from build123d import *

# Parameters (mm, degrees)
F0_R     = 16.6624
F1_DEPTH = 54.76875
F2_R     = 29.760102
F3_DEPTH = 20.6248
F4_R     = 11.1125
F5_DEPTH = 26.1874


with BuildPart() as f1:
    # F0 (on Top) → F1 (new body)
    with BuildSketch(Plane.XY):
        Circle(F0_R)
    extrude(amount=F1_DEPTH)

    # F2 (on face) → F3 (join)
    with BuildSketch(Plane(origin=(0, 0, 0), x_dir=(1, 0, 0), z_dir=(0, 0, -1))):
        Circle(F2_R)
    extrude(amount=F3_DEPTH)

    # F4 (on face) → F5 (join)
    with BuildSketch(Plane(origin=(0, 0, -20.6248), x_dir=(1, 0, 0), z_dir=(0, 0, -1))):
        Circle(F4_R)
    extrude(amount=F5_DEPTH)


solid = f1.part
Here's how the part is built. I have some questions about the finished solid (model axes, mm). A direction names the side the tool comes from. Round coordinates to 2 decimals unless told otherwise and drop trailing zeros. Order: outer loops, then holes, each group sorted by start corner. A loop starts at its lowest first (then second) coordinate and runs counter-clockwise, first axis right, second up. Notation, with made-up numbers: (8, -8) -> (21, -8) arc R21 cw to (21, 0) -> close; hole circle Ø1 at (0, 71.5). An arc over 180 degrees is marked (long way). Return JSON: item names as keys, results as strings.
Q1. If we section it at D-D on y = 13.5: List the corners of the cut face in (x, z) for me.
Filled sheet:
{"outline": "(-26.52, -20.62) -> (26.52, -20.62) -> (26.52, 0) -> (9.77, 0) -> (9.77, 54.77) -> (-9.77, 54.77) -> (-9.77, 0) -> (-26.52, 0) -> close"}
Q2. If we section it at A-A on x = 0: List the corners of the cut face in (y, z) for me, plus the area to 3 significant figures.
Filled sheet:
{"outline": "(-29.76, -20.62) -> (-11.11, -20.62) -> (-11.11, -46.81) -> (11.11, -46.81) -> (11.11, -20.62) -> (29.76, -20.62) -> (29.76, 0) -> (16.66, 0) -> (16.66, 54.77) -> (-16.66, 54.77) -> (-16.66, 0) -> (-29.76, 0) -> close", "area": "3,630 mm^2"}
Q3. Which directions (+Z, -Z, +X, -X, +Y, -Y) give clear straight access to the entire face, cutting with the end or side of a thin tool? Please do faces 1 (the cylindrical face through (15.893, 5.005, 27.001)), 2 (the flat face through (0, 0, -46.812)), 3 (the flat face through (0, 13, -20.625)).
Filled sheet:
{"face 1": "+Z", "face 2": "-Z, +X, -X, +Y, -Y", "face 3": "-Z"}
Q4. I need wall thicknesses on line 1 along Z through (x, y) = (26.5, 7.5); line 2 along Z through (x, y) = (3.5, 15.5); line 3 along Y through (x, z) = (-1, -15.5). Which ranges of each line are inside material? Lowest first, please. Write a range as from..to.
Filled sheet:
{"line 1": "z = -20.62..0", "line 2": "z = -20.62..54.77", "line 3": "y = -29.74..29.74"}
Q5. If we section it at C-C on z = 8: List the corners of the cut face in (x, y) for me.
Filled sheet:
{"outline": "circle Ø33.32 at (0, 0)"}
Q6. For pin 1 Ø12 at (x, y) = (21, -19) entering from -Z; pin 2 Ø5 at (x, z) = (9.5, 43) entering from -Y; pin 3 Ø1 at (x, z) = (-5, -16) entering from +Y; pin 4 Ø4 at (x, y) = (-11.5, 1) entering from -Z, each with a flat end and sliding along its axis, tell me the tip position at first contact or that it passes through.
Filled sheet:
{"pin 1": "stops at z = -20.62", "pin 2": "stops at y = -15.12", "pin 3": "stops at y = 29.42", "pin 4": "stops at z = -46.81"}
